```python
from build123d import *

# Parameters (mm, degrees)
PAD_DEPTH       = 58
SKETCH001_R     = 9.5
SKETCH001_R_2   = 7.6
PAD001_DEPTH    = 58
SKETCH002_R     = 7.6
SKETCH002_R_2   = 3
POCKET_DEPTH    = 58
SKETCH003_R     = 4.1
SKETCH003_W     = 9
SKETCH003_H     = 33
POCKET001_DEPTH = 55
SKETCH004_W     = 16
SKETCH004_H     = 13
POCKET002_DEPTH = 45
PAD002_DEPTH    = 58
SKETCH006_R     = 1.6
POCKET003_DEPTH = 17
SKETCH007_W     = 18
SKETCH007_H     = 58
POCKET004_DEPTH = 25
SKETCH008_W     = 17
SKETCH008_H     = 33
POCKET005_DEPTH = 5
SKETCH009_W     = 7
SKETCH009_H     = 33
POCKET006_DEPTH = 5
SKETCH010_W     = 8
SKETCH010_H     = 49
POCKET007_DEPTH = 45
SKETCH011_W     = 4
SKETCH011_H     = 17
POCKET008_DEPTH = 20
POCKET009_DEPTH = 58
FILLET_R        = 3
FILLET001_R     = 3


with BuildPart() as part:
    # Sketch → Pad (new body)
    with BuildSketch(Plane(origin=(-133, 0, 90), x_dir=(1, 0, 0), z_dir=(0, 0, 1))):
        Polygon((-47.676132, 21.976631), (5.323868, 21.976631), (5.323868, 5.976631), (-12.676132, 5.976631), (-12.676132, -0.023369), (-16.676132, -7.023369), (-24.676132, -7.023369), (-31.676132, 5.976631), (-47.676132, 5.976631), align=None)
    extrude(amount=PAD_DEPTH)

    # Sketch001 → Pad001 (new body)
    with BuildSketch(Plane(origin=(-133, 0, 148), x_dir=(1, 0, 0), z_dir=(0, 0, 1))):
        with Locations((-38.176132, -0.523369)):
            Circle(SKETCH001_R)
        with Locations((-38.176132, -0.523369)):
            Circle(SKETCH001_R_2, mode=Mode.SUBTRACT)
    extrude(amount=-PAD001_DEPTH)

    # Sketch002 → Pocket (cut)
    with BuildSketch(Plane(origin=(-133, 0, 148), x_dir=(1, 0, 0), z_dir=(0, 0, 1))):
        with Locations((-38.176132, -0.523369)):
            Circle(SKETCH002_R)
        with Locations((-21.176132, -0.523369)):
            Circle(SKETCH002_R_2)
    extrude(amount=-POCKET_DEPTH, mode=Mode.SUBTRACT)

    # Sketch003 → Pocket001 (cut)
    with BuildSketch(Plane(origin=(-180.676132, 0, 90), x_dir=(0, -1, 0), z_dir=(-1, 0, 0))):
        with Locations((-13.476631, 52)):
            Circle(SKETCH003_R)
        with Locations((-13.476631, 7)):
            Circle(SKETCH003_R)
        with Locations((-13.676631, 29.5)):
            Rectangle(SKETCH003_W, SKETCH003_H)
    extrude(amount=-POCKET001_DEPTH, mode=Mode.SUBTRACT)

    # Sketch004 → Pocket002 (cut)
    with BuildSketch(Plane(origin=(-133, 0, 148), x_dir=(1, 0, 0), z_dir=(0, 0, 1))):
        with Locations((-20.676132, -0.523369)):
            Rectangle(SKETCH004_W, SKETCH004_H)
    extrude(amount=-POCKET002_DEPTH, mode=Mode.SUBTRACT)

    # Sketch005 → Pad002 (new body)
    with BuildSketch(Plane(origin=(-133, 0, 148), x_dir=(1, 0, 0), z_dir=(0, 0, 1))):
        Polygon((-47.676132, 21.976631), (-91.676132, 21.976631), (-91.676132, 11.976631), (-81.676132, 11.976631), (-47.676132, 5.976631), align=None)
    extrude(amount=-PAD002_DEPTH)

    # Sketch006 → Pocket003 (cut)
    with BuildSketch(Plane(origin=(-133, 21.976631, 90), x_dir=(-1, 0, 0), z_dir=(0, 1, 0))):
        with Locations((56.676132, 44.5)):
            Circle(SKETCH006_R)
        with Locations((56.676132, 13.5)):
            Circle(SKETCH006_R)
        with Locations((87.676132, 13.5)):
            Circle(SKETCH006_R)
        Polygon((91.676132, 18), (81.676132, 18), (81.676132, 16), (59.676132, 16), (59.676132, 39), (61.676132, 39), (61.676132, 49), (47.676132, 49), (47.676132, 58), (91.676132, 58), align=None)
    extrude(amount=-POCKET003_DEPTH, mode=Mode.SUBTRACT)

    # Sketch007 → Pocket004 (cut)
    with BuildSketch(Plane(origin=(-133, 5.976631, 90), x_dir=(1, 0, 0), z_dir=(0, -1, 0))):
        with Locations((-3.676132, 29)):
            Rectangle(SKETCH007_W, SKETCH007_H)
    extrude(amount=-POCKET004_DEPTH, mode=Mode.SUBTRACT)

    # Sketch008 → Pocket005 (cut)
    with BuildSketch(Plane(origin=(-133, 21.976631, 90), x_dir=(-1, 0, 0), z_dir=(0, 1, 0))):
        with Locations((30.176132, 29.5)):
            Rectangle(SKETCH008_W, SKETCH008_H)
    extrude(amount=-POCKET005_DEPTH, mode=Mode.SUBTRACT)

    # Sketch009 → Pocket006 (cut)
    with BuildSketch(Plane(origin=(-133, 5.976631, 90), x_dir=(1, 0, 0), z_dir=(0, -1, 0))):
        with Locations((-25.176132, 29.5)):
            Rectangle(SKETCH009_W, SKETCH009_H)
    extrude(amount=-POCKET006_DEPTH, mode=Mode.SUBTRACT)

    # Sketch010 → Pocket007 (cut)
    with BuildSketch(Plane(origin=(-224.676132, 0, 90), x_dir=(0, -1, 0), z_dir=(-1, 0, 0))):
        with Locations((-9.976631, 24.5)):
            Rectangle(SKETCH010_W, SKETCH010_H)
    extrude(amount=-POCKET007_DEPTH, mode=Mode.SUBTRACT)

    # Sketch011 → Pocket008 (cut)
    with BuildSketch(Plane(origin=(-192.676132, 0, 90), x_dir=(0, -1, 0), z_dir=(-1, 0, 0))):
        with Locations((-15.976631, 27.5)):
            Rectangle(SKETCH011_W, SKETCH011_H)
    extrude(amount=-POCKET008_DEPTH, mode=Mode.SUBTRACT)

    # Sketch012 → Pocket009 (cut)
    with BuildSketch(Plane(origin=(-133, 0, 148), x_dir=(1, 0, 0), z_dir=(0, 0, 1))):
        Polygon((-38.722618, -1.360837), (-49.563332, 5.713227), (-49.016846, 6.550695), (-38.176132, -0.523369), align=None)
    extrude(amount=-POCKET009_DEPTH, mode=Mode.SUBTRACT)

    # Fillet
    fillet_edges = [part.edges().sort_by_distance(p)[0] for p in [
        (-224.676132, 17.976631, 108),
    ]]
    fillet(fillet_edges, radius=FILLET_R)

    # Fillet001
    fillet001_edges = [part.edges().sort_by_distance(p)[0] for p in [
        (-194.676132, 17.976631, 139),
    ]]
    fillet(fillet001_edges, radius=FILLET001_R)


solid = part.part
```
Design review of the part built by this model. Coordinates are the model's own, in mm. A direction names the side the tool comes from. Give positions to 0.01 mm unless a question says otherwise; leave off trailing zeros. Order: outer loops, then holes, each group sorted by start corner. A loop starts at its lowest first (then second) coordinate and runs counter-clockwise, first axis right, second up. Notation, with made-up numbers: (73.5, 50.25) -> (82.5, 50.25) arc R16 cw to (82.5, 73.25) -> close; hole circle Ø8 at (80.5, 85). An arc over 180 degrees is marked (long way). Write each question's results on one line, items separated by ' | '. Start each with the question number.
Q1. For pin 1 (5 mm diameter, centred on x = -165.5, z = 113.5, fed in from -Y); pin 2 (5.5 mm diameter, centred on x = -204.5, z = 104, fed in from -Y); pin 3 (2.5 mm diameter, centred on x = -220.68, z = 103.5, fed in from +Y) (3 decimals); pin 4 (9.5 mm diameter, centred on x = -184.5, z = 121.5, fed in from -Y), all flat-tipped, find the tip position at first contact; note any pin that passes through.
Q2. Add section D-D on y = 12. Give the boundary of the cut face in (x, z), and give its area (3 significant figures).
Q3. Add section B-B on y = 8. Give the boundary of the cut face in (x, z).
Q4. Machinability: for faces 5 (the flat face through (-194, 18, 129)), 6 (the flat face through (-154.676, 20, 119)), 7 (the flat face through (-161.676, 5, 126)), 8 (the flat face through (-152, 5.977, 130)), 9 (the flat face through (-187, 16, 109)), which of the approach directions +Z, -Z, +X, -X, +Y, -Y give a long, thin tool a straight path to every point of the face, cutting with its end or side? Answer none if there is none.
Q5. Add section C-C on z = 97. Give the boundary of the cut face in (x, y), and give its area (3 significant figures).
Q6. Wall thickness on L1, parallel to X at y = 17, z = 103.5; L2, parallel to Y at x = -154.5, z = 97; L3, parallel to X at y = 20.5, z = 109.5: over which ranges is each line inside the solid? List them lowest first. Write a range as from..to.
Q7. Mouldability with a two-part tool opening along Z and no side actions: class faces 1 (the flat face through (-154, -7.023, 96)), 2 (the flat face through (-218, 18, 108)), 3 (the flat face through (-177, 13, 90)), 4 (the flat face through (-187, 16, 126)) as +Z half, -Z half, draft (parallel to the pull), parting line (faces both ways), or undercut.
Q8. Add section A-A on z = 130.5. Give the boundary of the cut face in (x, y), and give its area (3 significant figures).
Found:
1) pin 1: stops at y = -9.48 | pin 2: stops at y = 13.98 | pin 3: passes through | pin 4: stops at y = -4.61
2) outline: (-180.68, 145.82) -> (-145.68, 145.82) -> (-145.68, 148) -> (-180.68, 148) -> close; (-179.68, 90) -> (-145.68, 90) -> (-145.68, 93.18) -> (-179.68, 93.18) -> close; (-179.68, 100.82) -> (-145.68, 100.82) -> (-145.68, 103) -> (-179.68, 103) -> close; (-179.68, 136) -> (-145.68, 136) -> (-145.68, 138.18) -> (-179.68, 138.18) -> close | area: 332 mm2
3) outline: (-180.68, 139) -> (-179.68, 139) -> (-179.68, 90) -> (-145.68, 90) -> (-145.68, 148) -> (-180.68, 148) -> close; hole (-161.68, 103) -> (-154.68, 103) -> (-154.68, 136) -> (-161.68, 136) -> close
4) face 5: -X, +Y, -Y | face 6: +Y, -Y | face 7: -Y | face 8: +Z, +X, -Y | face 9: +X, -X, -Y
5) outline: (-224.68, 13.98) -> (-180.68, 13.98) -> (-180.68, 17.58) -> (-145.68, 17.58) -> (-145.68, 21.98) -> (-224.68, 21.98) -> close; (-179.68, 5.98) -> (-178.1, 5.98) arc R9.5 ccw to (-179.13, 4.67) -> (-177.54, 3.63) arc R7.6 cw (long way) to (-178.03, 2.76) -> (-179.63, 3.8) arc R9.5 ccw (long way) to (-161.73, 0.51) -> (-157.68, -7.02) -> (-149.68, -7.02) -> (-145.68, -0.02) -> (-145.68, 9.38) -> (-179.68, 9.38) -> close; hole circle Ø6 at (-154.18, -0.52) | area: 849 mm2
6) L1: x = -224.68..-222.28, -219.08..-191.28, -188.08..-180.68 | L2: y = -7.02..-3.51, 2.46..9.38, 17.58..21.98 | L3: x = -192.68..-171.68, -154.68..-145.68
7) face 1: draft | face 2: +Z half | face 3: -Z half | face 4: undercut
8) outline: (-194.68, 13.98) -> (-180.68, 13.98) -> (-180.68, 18.18) -> (-171.68, 18.18) -> (-171.68, 21.98) -> (-194.68, 21.98) -> close; (-179.68, 5.98) -> (-178.1, 5.98) arc R9.5 ccw to (-179.13, 4.67) -> (-177.54, 3.63) arc R7.6 cw (long way) to (-178.03, 2.76) -> (-179.63, 3.8) arc R9.5 ccw (long way) to (-161.73, 0.51) -> (-161.68, 0.41) -> (-161.68, 9.18) -> (-179.68, 9.18) -> close; (-154.68, 5.98) -> (-145.68, 5.98) -> (-145.68, 9.18) -> (-154.68, 9.18) -> close; (-154.68, 18.18) -> (-145.68, 18.18) -> (-145.68, 21.98) -> (-154.68, 21.98) -> close | area: 343 mm2
